Geometry check sheet. Reference: the model listing, model coordinates, mm. Face numbers are marked on the shaded views. A direction names the side the tool comes from. Round coordinates to 2 decimals unless told otherwise and drop trailing zeros. Write each loop counter-clockwise with the first axis right and the second up, starting at its lowest first coordinate (ties: lowest second). Pieces come first, ordered by that corner, then holes. Notation, with made-up numbers: M 11,1 L 33,1 A31 cw 33,27 Z; hole C -2,48.5 d3. An arc over 180 degrees is marked long. Put each result on its own line as item: value. Start each with the question number.
(1) Material ranges on probe 1 along Y at (x, z) = (-24, 39); probe 2 along Z at (x, y) = (1.5, 7.5); probe 3 along Z at (x, y) = (41, 34), recorded low to high.
(2) Section check A-A on x = 0. Record the cut outline in (y, z).
(3) Tool access check on the marked faces 5 and 6. Record the directions out of +Z, -Z, +X, -X, +Y, -Y that give a thin tool (end or side, any length) a straight path to the whole face; none if there is none.
(4) Mould release check, pull along Y, two halves, no side actions. Record for the marked faces 1, 2, 3 and 4: pulls with the +Y half, pulls with the -Y half, needs draft (parallel to the pull), parting line crosses it, or undercut.
(5) Section check D-D on x = -12.5. Record the cut outline in (y, z), then the cut area to 3 significant figures.
(6) Gauge pin test, flat ends, axial feed: pin 1 (12 mm diameter, centred on x = -4, y = 23.5, fed in from -Z); pin 2 (7.5 mm diameter, centred on y = 15, z = 49.5, fed in from -X); pin 3 (3.5 mm diameter, centred on x = 29.34, z = 29.34, fed in from -Y). Record the tip position at first contact, or that the pin passes through.
(7) Section check C-C on y = 16.5. Record the cut outline in (x, z), then the cut area to 3 significant figures.
(8) Section check B-B on z = 0. Count the separate pieces of the cut face and the enclosed holes in it, then the cut area to 3 significant figures.
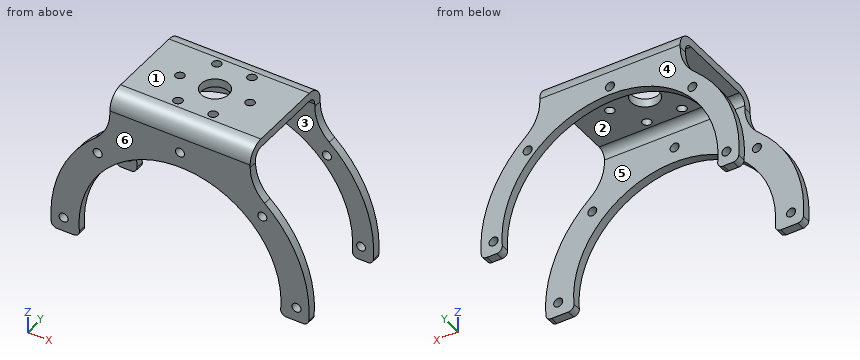
from build123d import *

# Parameters (mm, degrees)
SKETCH1_R                    = 1
BASE_FLANGE1_DEPTH           = 3
EDGE_FLANGE1_STRIP_W         = 18
EDGE_FLANGE1_STRIP_H         = 3
EDGE_FLANGE1_STRIP_CUT_DEPTH = 50
EDGE_FLANGE1_DEPTH           = 50
EDGE_FLANGE1_START           = 3
EDGE_FLANGE1_PROFILE_W       = 50
EDGE_FLANGE1_PROFILE_H       = 30
EDGE_FLANGE1_PROFILE_R       = 1
EDGE_FLANGE1_PROFILE_R_2     = 5
EDGE_FLANGE1_FLAT_DEPTH      = 3
EDGE_FLANGE2_STRIP_W         = 18
EDGE_FLANGE2_STRIP_H         = 3
EDGE_FLANGE2_STRIP_CUT_DEPTH = 50
EDGE_FLANGE2_DEPTH           = 50
EDGE_FLANGE2_START           = 3
EDGE_FLANGE2_PROFILE_R       = 1
EDGE_FLANGE2_FLAT_DEPTH      = 3
FILLET1_R                    = 15
FILLET2_R                    = 2
M3_CLEARANCE_HOLE1_D         = 3.2
M3_CLEARANCE_HOLE1_DEPTH     = 136
M3_CLEARANCE_HOLE1_TIP       = 0.96137699
M3_CLEARANCE_HOLE2_D         = 3.2
M3_CLEARANCE_HOLE2_DEPTH     = 136
M3_CLEARANCE_HOLE2_TIP       = 0.96137699


# Sheet-metal steps are written as plain solids
with BuildPart() as part:
    # Sketch1 → Base-Flange1 (new body)
    with BuildSketch(Plane(origin=(0, 0, 0), x_dir=(1, 0, 0), z_dir=(0, 1, 0))):
        with BuildLine():
            Line((-45.727453461, 5), (-35.65108694, 5))
            ThreePointArc((-35.65108694, 5), (0, -36), (35.65108694, 5))
            Line((35.65108694, 5), (45.727453461, 5))
            ThreePointArc((45.727453461, 5), (41.546682673, -19.745205972), (25, -38.613469153))
            Line((25, -38.613469153), (25, -50))
            Line((25, -50), (-25, -50))
            Line((-25, -50), (-25, -38.613469153))
            ThreePointArc((-25, -38.613469153), (-41.546682673, -19.745205972), (-45.727453461, 5))
        make_face()
        with Locations(Location((-41.5, 0, 0), (0, 0, 270))):
            Circle(SKETCH1_R, mode=Mode.SUBTRACT)
        with Locations(Location((41.5, 0, 0), (0, 0, 270))):
            Circle(SKETCH1_R, mode=Mode.SUBTRACT)
        with Locations(Location((-29.344931419, -29.344931419, 0), (0, 0, 270))):
            Circle(SKETCH1_R, mode=Mode.SUBTRACT)
        with Locations(Location((0, -41.5, 0), (0, 0, 270))):
            Circle(SKETCH1_R, mode=Mode.SUBTRACT)
        with Locations(Location((29.344931419, -29.344931419, 0), (0, 0, 270))):
            Circle(SKETCH1_R, mode=Mode.SUBTRACT)
    extrude(amount=-BASE_FLANGE1_DEPTH)

    # Edge-Flange1 strip (across the edge) → Edge-Flange1 strip cut (cut)
    with BuildSketch(Plane(origin=(-25, 0, 50), x_dir=(0, 0, -1), z_dir=(1, 0, 0))):
        with Locations((-6, -1.5)):
            Rectangle(EDGE_FLANGE1_STRIP_W, EDGE_FLANGE1_STRIP_H)
    extrude(amount=EDGE_FLANGE1_STRIP_CUT_DEPTH, mode=Mode.SUBTRACT)

    # Edge-Flange1 bend section (across the edge) → Edge-Flange1 (add)
    with BuildSketch(Plane(origin=(-25, 0, 50), x_dir=(0, 0, -1), z_dir=(1, 0, 0))):
        with BuildLine():
            Line((-3, 3), (0, 3))
            ThreePointArc((0, 3), (0.878679656, 0.878679656), (3, 0))
            Line((3, 0), (3, -3))
            ThreePointArc((3, -3), (-1.242640687, -1.242640687), (-3, 3))
        make_face()
    extrude(amount=EDGE_FLANGE1_DEPTH)

    # Edge-Flange1 profile (on flange) → Edge-Flange1 flat (add)
    with BuildSketch(Plane.XY.offset(50).offset(EDGE_FLANGE1_START)):
        with Locations((0, 18)):
            Rectangle(EDGE_FLANGE1_PROFILE_W, EDGE_FLANGE1_PROFILE_H)
        with Locations((-6.25, 5.674682453)):
            Circle(EDGE_FLANGE1_PROFILE_R, mode=Mode.SUBTRACT)
        with Locations((-12.5, 16.5)):
            Circle(EDGE_FLANGE1_PROFILE_R, mode=Mode.SUBTRACT)
        with Locations((6.25, 5.674682453)):
            Circle(EDGE_FLANGE1_PROFILE_R, mode=Mode.SUBTRACT)
        with Locations((0, 16.5)):
            Circle(EDGE_FLANGE1_PROFILE_R_2, mode=Mode.SUBTRACT)
        with Locations((-6.25, 27.325317547)):
            Circle(EDGE_FLANGE1_PROFILE_R, mode=Mode.SUBTRACT)
        with Locations((12.5, 16.5)):
            Circle(EDGE_FLANGE1_PROFILE_R, mode=Mode.SUBTRACT)
        with Locations((6.25, 27.325317547)):
            Circle(EDGE_FLANGE1_PROFILE_R, mode=Mode.SUBTRACT)
    extrude(amount=-EDGE_FLANGE1_FLAT_DEPTH)

    # Edge-Flange2 strip (across the edge) → Edge-Flange2 strip cut (cut)
    with BuildSketch(Plane(origin=(-25, 33, 50), x_dir=(0, -1, 0), z_dir=(1, 0, 0))):
        with Locations((-6, -1.5)):
            Rectangle(EDGE_FLANGE2_STRIP_W, EDGE_FLANGE2_STRIP_H)
    extrude(amount=EDGE_FLANGE2_STRIP_CUT_DEPTH, mode=Mode.SUBTRACT)

    # Edge-Flange2 bend section (across the edge) → Edge-Flange2 (add)
    with BuildSketch(Plane(origin=(-25, 33, 50), x_dir=(0, -1, 0), z_dir=(1, 0, 0))):
        with BuildLine():
            Line((-3, 3), (0, 3))
            ThreePointArc((0, 3), (0.878679656, 0.878679656), (3, 0))
            Line((3, 0), (3, -3))
            ThreePointArc((3, -3), (-1.242640687, -1.242640687), (-3, 3))
        make_face()
    extrude(amount=EDGE_FLANGE2_DEPTH)

    # Edge-Flange2 profile (on flange) → Edge-Flange2 flat (add)
    with BuildSketch(Plane(origin=(0, 33, 50), x_dir=(1, 0, 0), z_dir=(0, 1, 0)).offset(EDGE_FLANGE2_START)):
        with BuildLine():
            ThreePointArc((25, 11.386530847), (41.546682673, 30.254794028), (45.727453461, 55))
            Line((45.727453461, 55), (38.173943993, 55))
            ThreePointArc((38.173943993, 55), (0, 11.5), (-38.173943993, 55))
            Line((-38.173943993, 55), (-45.727453461, 55))
            ThreePointArc((-45.727453461, 55), (-41.546682673, 30.254794028), (-25, 11.386530847))
            Line((-25, 11.386530847), (-25, 3))
            Line((-25, 3), (25, 3))
            Line((25, 3), (25, 11.386530847))
        make_face()
        with Locations((29.35734241, 20.64265759)):
            Circle(EDGE_FLANGE2_PROFILE_R, mode=Mode.SUBTRACT)
        with Locations((0, 8.482448208)):
            Circle(EDGE_FLANGE2_PROFILE_R, mode=Mode.SUBTRACT)
        with Locations((-29.35734241, 20.64265759)):
            Circle(EDGE_FLANGE2_PROFILE_R, mode=Mode.SUBTRACT)
        with Locations((41.517551792, 50)):
            Circle(EDGE_FLANGE2_PROFILE_R, mode=Mode.SUBTRACT)
        with Locations((-41.517551792, 50)):
            Circle(EDGE_FLANGE2_PROFILE_R, mode=Mode.SUBTRACT)
    extrude(amount=-EDGE_FLANGE2_FLAT_DEPTH)

    # Fillet1
    fillet1_edges = [part.edges().sort_by_distance(p)[0] for p in [
        (-25, 34.5, 38.613469153),
        (25, 34.5, 38.613469153),
        (25, -1.5, 38.613469153),
        (-25, -1.5, 38.613469153),
    ]]
    fillet(fillet1_edges, radius=FILLET1_R)

    # Fillet2
    fillet2_edges = [part.edges().sort_by_distance(p)[0] for p in [
        (45.727453461, 34.5, -5),
        (38.173943993, 34.5, -5),
        (-38.173943993, 34.5, -5),
        (-45.727453461, 34.5, -5),
        (-45.727453461, -1.5, -5),
        (-35.65108694, -1.5, -5),
        (35.65108694, -1.5, -5),
        (45.727453461, -1.5, -5),
    ]]
    fillet(fillet2_edges, radius=FILLET2_R)

    # M3 Clearance Hole1
    with Locations(Plane(origin=(0, -3, 0), x_dir=(-1, 0, 0), z_dir=(0, -1, 0))):
        with Locations((41.5, 0), (29.344931419, -29.344931419), (0, -41.5), (-29.344931419, -29.344931419), (-41.5, 0)):
            Hole(M3_CLEARANCE_HOLE1_D / 2, depth=M3_CLEARANCE_HOLE1_DEPTH)
            with Locations((0, 0, -(M3_CLEARANCE_HOLE1_DEPTH + M3_CLEARANCE_HOLE1_TIP / 2))):  # 118° drill point
                Cone(0, M3_CLEARANCE_HOLE1_D / 2, M3_CLEARANCE_HOLE1_TIP, mode=Mode.SUBTRACT)

    # M3 Clearance Hole2
    with Locations(Plane(origin=(0, 0, 50), x_dir=(-1, 0, 0), z_dir=(0, 0, -1))):
        with Locations((6.25, 27.325317547), (12.5, 16.5), (6.25, 5.674682453), (-6.25, 5.674682453), (-12.5, 16.5), (-6.25, 27.325317547)):
            Hole(M3_CLEARANCE_HOLE2_D / 2, depth=M3_CLEARANCE_HOLE2_DEPTH)
            with Locations((0, 0, -(M3_CLEARANCE_HOLE2_DEPTH + M3_CLEARANCE_HOLE2_TIP / 2))):  # 118° drill point
                Cone(0, M3_CLEARANCE_HOLE2_D / 2, M3_CLEARANCE_HOLE2_TIP, mode=Mode.SUBTRACT)


solid = part.part
Answers follow:
1. probe 1: y = -3 to 0, 33 to 36
1. probe 2: z = 50 to 53
1. probe 3: z = -5 to -1.52, 1.52 to 20.86
2. outline: M -3,36 L 0,36 L 0,39.9 L -3,39.9 Z; M -3,43.1 L 0,43.1 L 0,47 A3 cw 3,50 L 11.5,50 L 11.5,53 L 3,53 A6 ccw -3,47 Z; M 21.5,50 L 30,50 A3 cw 33,47 L 33,43.1 L 36,43.1 L 36,47 A6 ccw 30,53 L 21.5,53 Z; M 33,38.5 L 36,38.5 L 36,39.9 L 33,39.9 Z
3. face 5: -Z, +X, -X
3. face 6: +Z, -Z, +X, -X, -Y
4. face 1: needs draft
4. face 2: undercut
4. face 3: undercut
4. face 4: pulls with the +Y half
5. outline: M -3,33.76 L 0,33.76 L 0,47 A3 cw 3,50 L 14.9,50 L 14.9,53 L 3,53 A6 ccw -3,47 Z; M 18.1,50 L 30,50 A3 cw 33,47 L 33,36.41 L 36,36.41 L 36,47 A6 ccw 30,53 L 18.1,53 Z
5. area: 185 mm^2
6. pin 1: stops at z = 50
6. pin 2: stops at x = -25
6. pin 3: stops at y = -3
7. outline: M -25,50 L -14.1,50 L -14.1,53 L -25,53 Z; M -10.9,50 L -5,50 L -5,53 L -10.9,53 Z; M 5,50 L 10.9,50 L 10.9,53 L 5,53 Z; M 14.1,50 L 25,50 L 25,53 L 14.1,53 Z
7. area: 101 mm^2
8. separate pieces: 8
8. enclosed holes: 0
8. area: 66.6 mm^2
